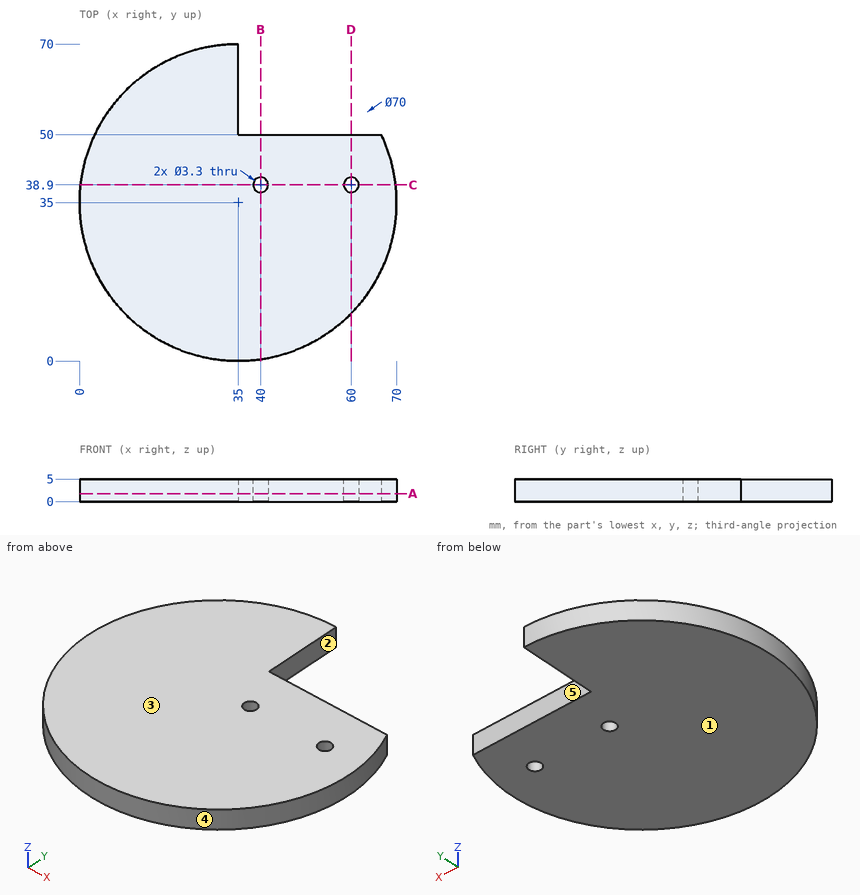
Drawing for the job (mm, zero at the part's lowest x, y, z). A direction names the side the tool comes from. Coordinates: 2 decimals unless noted, no trailing zeros. Write each loop counter-clockwise with the first axis right and the second up, starting at its lowest first coordinate (ties: lowest second). Pieces come first, ordered by that corner, then holes. Notation, with made-up numbers: (33, 20.25) - (91, 20.25) arc R22 cw to (91, 38.25) - close; hole circle Ø4 at (19, -7). An arc over 180 degrees is marked (long way). Write each question's results on one line, items separated by ' | '. Start each with the question number.
1) Flat gauge pins, fed straight in: P1, Ø2.5, axis at y = 55.5, z = 2, coming from the +X side; P2, Ø2, axis at y = 15, z = 1.5, coming from the +X side; P3, Ø3, axis at x = 10, z = 3, coming from the -Y side. Where does each tip first touch, or does it go through?
2) Mould opens along Z. For the marked faces 1, 2 and 3 say: pulls with the +Z half, pulls with the -Z half, needs draft (parallel to the pull), parting line crosses it, or undercut.
3) Cut at A-A (z = 1.75). Write the cut outline in (x, y), then the cut area to 3 significant figures.
4) Probe line 1 along Y through (x, z) = (60, 3.95); line 2 along X through (y, z) = (20.5, 1.4); line 3 along Y through (x, z) = (40, 2.55). List the from-to ranges inside material, lowest first. Write a range as from..to.
5) Cut at C-C (y = 38.9). Write the cut outline in (x, z), then the cut area to 3 significant figures.
6) Cut at B-B (x = 40). Write the cut outline in (y, z).
7) Cut at D-D (x = 60). Write the cut outline in (y, z).
8) 3-axis set-ups, long thin cutter, end or side, ignore diameter. For the marked faces 4 and 5: which of +Z, -Z, +X, -X, +Y, -Y reach the whole face in a straight line?
Returned:
1) P1: x = 35 | P2: x = 64.39 | P3: y = 9.06
2) face 1: pulls with the -Z half | face 2: needs draft | face 3: pulls with the +Z half
3) outline: (35, 50) - (35, 70) arc R35 ccw (long way) to (66.62, 50) - close; hole circle Ø3.3 at (40, 38.9); hole circle Ø3.3 at (60, 38.9) | area: 3,380 mm^2
4) line 1: 10.51..37.25, 40.55..50 | line 2: 3.14..66.86 | line 3: 0.36..37.25, 40.55..50
5) outline: (0.22, 0) - (38.35, 0) - (38.35, 5) - (0.22, 5) - close; (41.65, 0) - (58.35, 0) - (58.35, 5) - (41.65, 5) - close; (61.65, 0) - (69.78, 0) - (69.78, 5) - (61.65, 5) - close | area: 315 mm^2
6) outline: (0.36, 0) - (37.25, 0) - (37.25, 5) - (0.36, 5) - close; (40.55, 0) - (50, 0) - (50, 5) - (40.55, 5) - close
7) outline: (10.51, 0) - (37.25, 0) - (37.25, 5) - (10.51, 5) - close; (40.55, 0) - (50, 0) - (50, 5) - (40.55, 5) - close
8) face 4: +Z, -Z | face 5: +Z, -Z, +X, +Y
